The figure shows three views and two pictorial views of one solid part (mm, origin at its lowest corner). Answer the questions. A direction names the side the tool comes from. Give positions to 0.01 mm unless a question says otherwise; leave off trailing zeros. Order: outer loops, then holes, each group sorted by start corner. A loop starts at its lowest first (then second) coordinate and runs counter-clockwise, first axis right, second up. Notation, with made-up numbers: (-14, 49) -> (-9, 49) arc R14 cw to (-9, 75) -> close; hole circle Ø9 at (-37.5, 55). An arc over 180 degrees is marked (long way). One line per item, written item: value. Start each with the question number.
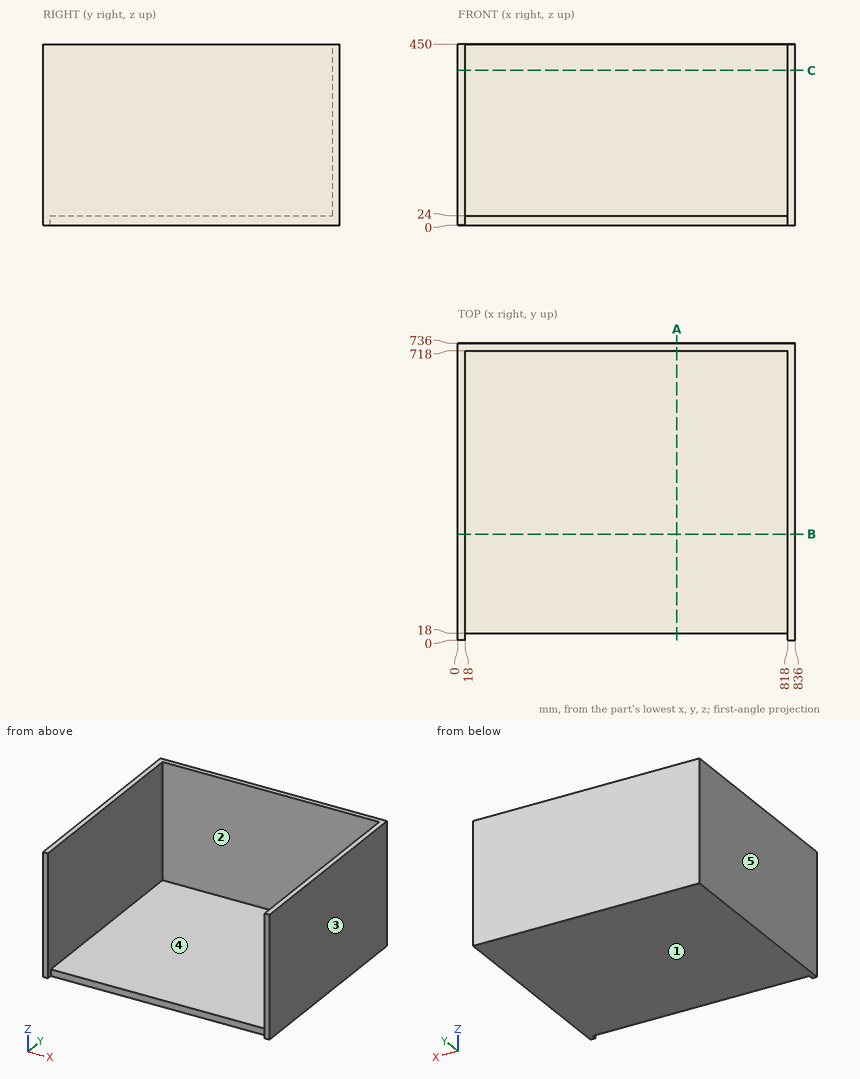
Item 1: Find section A-A on x = 543. Write down the section's boundary in (y, z), then the cut area to 3 significant figures.
Item 2: Find section C-C on z = 384.5. Write down the section's boundary in (x, y).
Item 3: A tool of negligible diameter and unlimited length cuts with its end or side. For the marked faces 1 and 2, from which of +Z, -Z, +X, -X, +Y, -Y can it reach the whole face along a straight path? Write none if from no direction.
Item 4: For a pull along X with two mould halves and no side action, classify the marked faces 3, 4 and 5 as +X half, -X half, draft (parallel to the pull), parting line (faces both ways), or undercut.
Item 5: Flat-ended cylindrical pins translate along their axes: pin 1 (1.5 mm diameter, centred on x = 571, y = 335.5, fed in from +Z); pin 2 (19 mm diameter, centred on x = 336.5, z = 14.5, fed in from -Y). Find the tip coordinate at first contact, or state that the pin passes through.
Item 6: Find the intervals of material crossed by line 1 (X direction, y = 465, z = 408.5); line 2 (Z direction, x = 720, y = 111.5); line 3 (Y direction, x = 721, z = 292.5), in increasing order. Write a range as from..to.
Item 7: Find section B-B on y = 263. Write down the section's boundary in (x, z).
Checks:
1. outline: (18, 0) -> (736, 0) -> (736, 450) -> (718, 450) -> (718, 24) -> (18, 24) -> close
1. area: 24,900 mm2
2. outline: (0, 0) -> (18, 0) -> (18, 718) -> (818, 718) -> (818, 0) -> (836, 0) -> (836, 736) -> (0, 736) -> close
3. face 1: -Z, +X, -X, +Y, -Y
3. face 2: +Z, -Y
4. face 3: +X half
4. face 4: undercut
4. face 5: -X half
5. pin 1: z = 24
5. pin 2: y = 18
6. line 1: 0..18, 818..836
6. line 2: 0..24
6. line 3: 718..736
7. outline: (0, 0) -> (836, 0) -> (836, 450) -> (818, 450) -> (818, 24) -> (18, 24) -> (18, 450) -> (0, 450) -> close
